Can you work these out from the model? Positions are in its coordinate system, mm. Face numbers are marked on the shaded views. A direction names the side the tool comes from. Coordinates: 2 decimals unless noted, no trailing zeros. Order: outer loops, then holes, each group sorted by start corner. A loop starts at its lowest first (then second) coordinate and runs counter-clockwise, first axis right, second up.
```python
from build123d import *

# Parameters (mm, degrees)
F1_DEPTH = 250
F2_DEPTH = 5


with BuildPart() as f1:
    # F0 (on Front) → F1 (new body)
    with BuildSketch(Plane.XZ):
        Polygon((-90, 220), (-125, 155), (-125, -145), (-65, -220), (65, -220), (125, -145), (125, 145), (90, 220), align=None)
    extrude(amount=F1_DEPTH)

    # F0 (on Front) → F2 (join)
    with BuildSketch(Plane.XZ):
        with BuildLine():
            Line((-125, -145), (-125, 155))
            Line((-125, 155), (-90, 220))
            Line((-90, 220), (90, 220))
            Line((90, 220), (125, 145))
            Line((125, 145), (125, -145))
            Line((125, -145), (150, -113.75))
            Line((150, -113.75), (150, 145))
            ThreePointArc((150, 145), (149.055004, 151.808581), (146.291458, 158.102436))
            Line((146.291458, 158.102436), (111.291458, 233.102436))
            ThreePointArc((111.291458, 233.102436), (102.195063, 241.82385), (90, 245))
            Line((90, 245), (-90, 245))
            ThreePointArc((-90, 245), (-102.195063, 241.82385), (-111.291458, 233.102436))
            Line((-111.291458, 233.102436), (-146.291458, 168.102436))
            ThreePointArc((-146.291458, 168.102436), (-149.055004, 161.808581), (-150, 155))
            Line((-150, 155), (-150, -113.75))
            Line((-150, -113.75), (-125, -145))
        make_face()
    extrude(amount=F2_DEPTH)


solid = f1.part
```
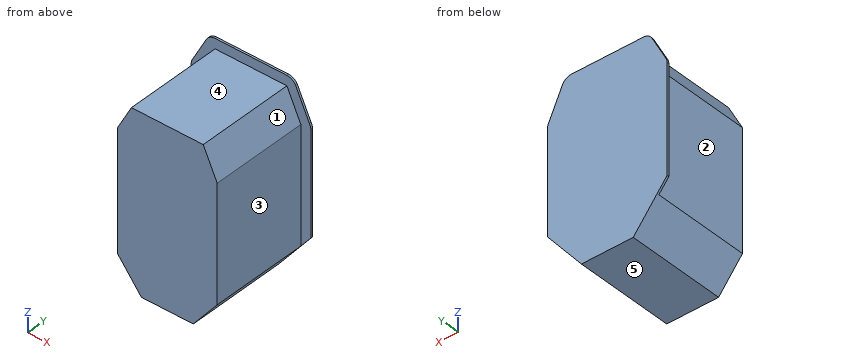
1. Imagine slicing it at C-C on x = 75. Please give me the cut outline in (y, z).
Completed:
outline: (-250, -207.5) - (0, -207.5) - (0, 245) - (-5, 245) - (-5, 220) - (-250, 220) - close
2. Please list where these lines run through material, in increasing order: probe 1 along Z at (x, y) = (19, -182); probe 2 along X at (y, z) = (-153, -140.5); probe 3 along Y at (x, z) = (122, 206.5).
Completed:
probe 1: z = -220 to 220
probe 2: x = -125 to 125
probe 3: y = -5 to 0
3. I'm going to push flat-ended pins straight in: pin 1 (10 mm diameter, centred on x = -54.5, z = 134.5, fed in from +Y); pin 2 (6 mm diameter, centred on y = -116.5, z = -120.5, fed in from -X); pin 3 (8 mm diameter, centred on y = -74.5, z = 102.5, fed in from +X); pin 4 (10 mm diameter, centred on x = 103.5, y = -187.5, fed in from -Z) (3 decimals). Where does each tip first touch, or does it pass through?
Completed:
pin 1: stops at y = 0
pin 2: stops at x = -125
pin 3: stops at x = 125
pin 4: stops at z = -178.125
4. Imagine slicing it at A-A on y = -219.5. Please give me the cut outline in (x, z).
Completed:
outline: (-125, -145) - (-65, -220) - (65, -220) - (125, -145) - (125, 145) - (90, 220) - (-90, 220) - (-125, 155) - close
5. On a 3-axis mill with a long thin cutter (end or side, diameter ignored), from which of +Z, -Z, +X, -X, +Y, -Y can I reach the whole of each face in a straight line? I mean the marked faces 1, 2, 3, 4 and 5. Say none if no direction works.
Completed:
face 1: +Z, +X, -Y
face 2: +Z, -Z, -X, -Y
face 3: +Z, -Z, +X, -Y
face 4: +Z, +X, -X, -Y
face 5: -Z, +X, -X, +Y, -Y
6. Imagine slicing it at D-D on x = 35. Please give me the cut outline in (y, z), then the cut area to 3 significant figures.
Completed:
outline: (-250, -220) - (0, -220) - (0, 245) - (-5, 245) - (-5, 220) - (-250, 220) - close
area: 110,000 mm2
7. Imagine slicing it at B-B on z = -123. Please give me the cut outline in (x, y), then the cut area to 3 significant figures.
Completed:
outline: (-142.6, -5) - (-125, -5) - (-125, -250) - (125, -250) - (125, -5) - (142.6, -5) - (142.6, 0) - (-142.6, 0) - close
area: 62,700 mm2
